```python
from build123d import *

# Parameters (mm, degrees)
SKETCH1_W           = 50
SKETCH1_H           = 60
SKETCH1_W_2         = 47
SKETCH1_H_2         = 57
BOSS_EXTRUDE6_DEPTH = 40
SKETCH7_W           = 50
SKETCH7_H           = 60
BOSS_EXTRUDE8_DEPTH = 1.5
SKETCH8_W           = 10
SKETCH8_H           = 2
BOSS_EXTRUDE9_DEPTH = 50
SKETCH9_R           = 1.55
CUT_EXTRUDE1_DEPTH  = 3


with BuildPart() as part:
    # Sketch1 → Boss-Extrude6 (new body)
    with BuildSketch(Plane(origin=(0, 0, 0), x_dir=(1, 0, 0), z_dir=(0, 1, 0))):
        Rectangle(SKETCH1_W, SKETCH1_H)
        Rectangle(SKETCH1_W_2, SKETCH1_H_2, mode=Mode.SUBTRACT)
    extrude(amount=BOSS_EXTRUDE6_DEPTH)

    # Sketch7 → Boss-Extrude8 (add)
    with BuildSketch(Plane.XZ):
        Rectangle(SKETCH7_W, SKETCH7_H)
    extrude(amount=BOSS_EXTRUDE8_DEPTH)

    # Sketch8 → Boss-Extrude9 (add)
    with BuildSketch(Plane(origin=(25, 0, 0), x_dir=(0, 0, -1), z_dir=(1, 0, 0))):
        with Locations((-35, 39)):
            Rectangle(SKETCH8_W, SKETCH8_H)
        with Locations((35, 39)):
            Rectangle(SKETCH8_W, SKETCH8_H)
    extrude(amount=-BOSS_EXTRUDE9_DEPTH)

    # Sketch9 → Cut-Extrude1 (cut)
    with BuildSketch(Plane(origin=(0, 40, 0), x_dir=(1, 0, 0), z_dir=(0, 1, 0))):
        with Locations(Location((-20, 35, 0), (0, 0, 270))):
            Circle(SKETCH9_R)
        with Locations(Location((20, 35, 0), (0, 0, 270))):
            Circle(SKETCH9_R)
        with Locations(Location((20, -35, 0), (0, 0, 270))):
            Circle(SKETCH9_R)
        with Locations(Location((-20, -35, 0), (0, 0, 270))):
            Circle(SKETCH9_R)
    extrude(amount=-CUT_EXTRUDE1_DEPTH, mode=Mode.SUBTRACT)


solid = part.part
```
Work out the finished part from the listing and answer in its coordinate system (mm). A direction names the side the tool comes from. Round coordinates to 2 decimals unless told otherwise and drop trailing zeros. Write each loop counter-clockwise with the first axis right and the second up, starting at its lowest first coordinate (ties: lowest second). Pieces come first, ordered by that corner, then holes. Notation, with made-up numbers: (21.25, -25.5) - (30.25, -25.5) arc R20 cw to (30.25, -13.5) - close; hole circle Ø6 at (41.25, 72.5). An arc over 180 degrees is marked (long way). Return JSON: item names as keys, results as strings. Group by question number.
Q1. The part is cut by section D-D on z = -6.5. Write down the section's boundary in (x, y).
Q2. The part is cut by section A-A on z = 35. Write down the section's boundary in (x, y), then the cut area to 3 significant figures.
Q3. Each of these flat-tipped pins is pushed along its axis until it touches: pin 1 Ø3 at (x, z) = (20, -35) entering from +Y; pin 2 Ø14 at (x, z) = (11, -10) entering from +Y; pin 3 Ø8 at (x, z) = (7.5, 36) entering from -Y; pin 4 Ø12 at (x, y) = (1.5, 25.5) entering from -Z. Where does it stop, or does it pass through?
Q4. The part is cut by section B-B on x = -20. Write down the section's boundary in (y, z).
Q5. The part is cut by section C-C on y = 10.5. Write down the section's boundary in (x, z).
Q6. Find the intervals of material crossed by L1, parallel to X at y = 38.6, z = -35; L2, parallel to X at y = 35, z = 4.5; L3, parallel to Z at x = -12.5, y = 26, in increasing order.
Q7. For faces 1 (the flat face through (-23.5, 20, 0)), 2 (the flat face through (0, 19, 30)), 3 (the flat face through (0, 38, -35)), determine the directions among +Z, -Z, +X, -X, +Y, -Y from which every point of the face is accessible in a straight line to the end or side of a thin tool.
Q8. The mould has two halves that part along Z. Classify faces 4 (the cylindrical face through (-18.69, 39.01, -34.17)), 5 (the flat face through (0, 19, -30)), 6 (the flat face through (25, 20, 1)), 7 (the flat face through (0, 39, 40)): released by +Z, released by -Z, zero draft, split by the parting line, or undercut.
Solved:
{
 "1": {"outline": "(-25, -1.5) - (25, -1.5) - (25, 40) - (23.5, 40) - (23.5, 0) - (-23.5, 0) - (-23.5, 40) - (-25, 40) - close"},
 "2": {"outline": "(-25, 38) - (-21.55, 38) - (-21.55, 40) - (-25, 40) - close; (-18.45, 38) - (18.45, 38) - (18.45, 40) - (-18.45, 40) - close; (21.55, 38) - (25, 38) - (25, 40) - (21.55, 40) - close", "area": "87.6 mm²"},
 "3": {"pin 1": "through", "pin 2": "y = 0", "pin 3": "y = 38", "pin 4": "z = -30"},
 "4": {"outline": "(-1.5, -30) - (38, -30) - (38, -33.45) - (40, -33.45) - (40, -28.5) - (0, -28.5) - (0, 28.5) - (40, 28.5) - (40, 33.45) - (38, 33.45) - (38, 30) - (-1.5, 30) - close; (38, -40) - (40, -40) - (40, -36.55) - (38, -36.55) - close; (38, 36.55) - (40, 36.55) - (40, 40) - (38, 40) - close"},
 "5": {"outline": "(-25, -30) - (25, -30) - (25, 30) - (-25, 30) - close; hole (-23.5, -28.5) - (23.5, -28.5) - (23.5, 28.5) - (-23.5, 28.5) - close"},
 "6": {"L1": "-25 to -21.55, -18.45 to 18.45, 21.55 to 25", "L2": "-25 to -23.5, 23.5 to 25", "L3": "-30 to -28.5, 28.5 to 30"},
 "7": {"face 1": "+Y", "face 2": "+Z, +X, -X, -Y", "face 3": "-Z, +X, -X, -Y"},
 "8": {"face 4": "undercut", "face 5": "released by -Z", "face 6": "zero draft", "face 7": "released by +Z"}
}
